Drawing for the job (mm, zero at the part's lowest x, y, z). Round coordinates to 2 decimals unless told otherwise and drop trailing zeros. Write each loop counter-clockwise with the first axis right and the second up, starting at its lowest first coordinate (ties: lowest second). Pieces come first, ordered by that corner, then holes. Notation, with made-up numbers: M 46.5,84.5 L 69.5,84.5 A27 ccw 69.5,108.5 Z; hole C 54,-29.5 d10. An arc over 180 degrees is marked long. Use a Markdown table: item, result.
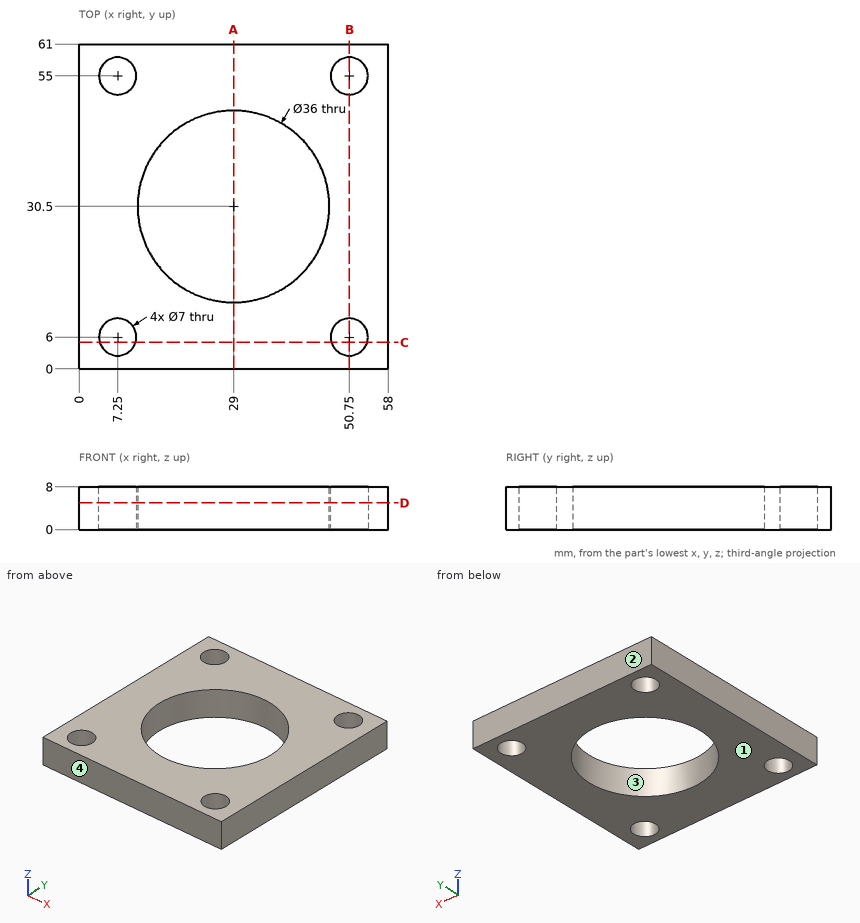
Q1. Cut at B-B on x = 50.75. Give the cut face in (y, z), and give its area (3 significant figures).
Response values:
| item | result |
|---|---|
| outline | M 0,0 L 2.5,0 L 2.5,8 L 0,8 Z; M 9.5,0 L 51.5,0 L 51.5,8 L 9.5,8 Z; M 58.5,0 L 61,0 L 61,8 L 58.5,8 Z |
| area | 376 mm2 |
Q2. Drill centre lines: L1, parallel to Y at x = 7.25, z = 5.5; L2, parallel to X at y = 4, z = 1; L3, parallel to X at y = 9, z = 7. Where is each one in solid material? Low to high.
Response values:
| item | result |
|---|---|
| L1 | y = 0 to 2.5, 9.5 to 51.5, 58.5 to 61 |
| L2 | x = 0 to 4.38, 10.12 to 47.88, 53.62 to 58 |
| L3 | x = 0 to 5.45, 9.05 to 48.95, 52.55 to 58 |
Q3. Cut at C-C on y = 5. Give the cut face in (x, z).
Response values:
| item | result |
|---|---|
| outline | M 0,0 L 3.9,0 L 3.9,8 L 0,8 Z; M 10.6,0 L 47.4,0 L 47.4,8 L 10.6,8 Z; M 54.1,0 L 58,0 L 58,8 L 54.1,8 Z |
Q4. Two-plate mould, pull along Y, no slides. Class the marked faces 1, 2, 3 and 4: +Y half, -Y half, draft (parallel to the pull), parting line (faces both ways), or undercut.
Response values:
| item | result |
|---|---|
| face 1 | draft |
| face 2 | +Y half |
| face 3 | undercut |
| face 4 | -Y half |
Q5. Drop flat-ended pins along their axis: P1, Ø11, axis at x = 7.25, y = 6, coming from the -Z side; P2, Ø4, axis at x = 7.25, y = 55, coming from the -Z side. Give the stop position or say it passes through.
Response values:
| item | result |
|---|---|
| P1 | stops at z = 0 |
| P2 | passes through |
Q6. Cut at A-A on x = 29. Give the cut face in (y, z).
Response values:
| item | result |
|---|---|
| outline | M 0,0 L 12.5,0 L 12.5,8 L 0,8 Z; M 48.5,0 L 61,0 L 61,8 L 48.5,8 Z |
Q7. Cut at D-D on z = 5. Give the cut face in (x, y), and give its area (3 significant figures).
Response values:
| item | result |
|---|---|
| outline | M 0,0 L 58,0 L 58,61 L 0,61 Z; hole C 7.25,6 d7; hole C 7.25,55 d7; hole C 29,30.5 d36; hole C 50.75,6 d7; hole C 50.75,55 d7 |
| area | 2,370 mm2 |
